Geometry check sheet. Reference: the model listing, model coordinates, mm. Round coordinates to 2 decimals unless told otherwise and drop trailing zeros. Write each loop counter-clockwise with the first axis right and the second up, starting at its lowest first coordinate (ties: lowest second). Pieces come first, ordered by that corner, then holes. Notation, with made-up numbers: (85, 61) -> (110, 61) arc R26 cw to (110, 90) -> close; hole circle Ø3 at (58.25, 49.25). An arc over 180 degrees is marked (long way). Put each result on its own line as item: value. Start each with the question number.
from build123d import *

# Parameters (mm, degrees)
F0_R     = 78.74
F1_DEPTH = 386.08
F3_D     = 10.8
F3_DEPTH = 38.1
F3_TIP   = 3.2446473427
F4_R     = 5.08
F5_R     = 7.62


with BuildPart() as f1:
    # F0 (on Front) → F1 (new body)
    with BuildSketch(Plane.XZ):
        Circle(F0_R)
    extrude(amount=F1_DEPTH)

    # F3
    with Locations(Plane.XZ.offset(386.08)):
        with Locations((0, 0)):
            Hole(F3_D / 2, depth=F3_DEPTH)
            with Locations((0, 0, -(F3_DEPTH + F3_TIP / 2))):  # 118° drill point
                Cone(0, F3_D / 2, F3_TIP, mode=Mode.SUBTRACT)

    # F4
    f4_edges = [f1.edges().sort_by_distance(p)[0] for p in [
        (-78.74, -386.08, 0),
    ]]
    fillet(f4_edges, radius=F4_R)

    # F5
    f5_edges = [f1.edges().sort_by_distance(p)[0] for p in [
        (-78.74, 0, 0),
    ]]
    fillet(f5_edges, radius=F5_R)


solid = f1.part
(1) Go/stop test with flat-tipped pins: pin 1 Ø4 at (x, y) = (-15.5, -145) entering from +Z; pin 2 Ø10 at (y, z) = (-270, -53.5) entering from -X; pin 3 Ø12 at (y, z) = (-268, -22) entering from -X. Record where each tip stops, or that it passes through.
(2) Material ranges on L1, parallel to Z at x = 0, y = -359.5; L2, parallel to X at y = -276, z = -43; L3, parallel to Z at x = -1.5, y = -188, recorded low to high. Write a range as from..to.
(3) Mould release check, pull along Z, two halves, no side actions. Record for faces 1 (the cylindrical face through (1.17, -366.76, -5.27)), 2 (the cylindrical face through (-62.485, -191.696, -47.912)), 3 (the flat face through (15, -386.08, 1)): +Z half, -Z half, draft (parallel to the pull), parting line (faces both ways), or undercut.
(4) Sectioned sample at A-A (y = -325.5). Record the cut outline in (x, z), and give its area (3 significant figures).
Found:
1. pin 1: z = 77.57
1. pin 2: x = -62.03
1. pin 3: x = -77.1
2. L1: -78.74..-5.4, 5.4..78.74
2. L2: -65.96..65.96
2. L3: -78.73..78.73
3. face 1: undercut
3. face 2: parting line
3. face 3: draft
4. outline: circle Ø157.48 at (0, 0)
4. area: 19,500 mm2
